Input: dimensioned drawing with shaded views. Units: mm. Origin: part minimum x, y, z. Give positions to 0.01 mm unless a question says otherwise; leave off trailing zeros. Write each loop counter-clockwise with the first axis right and the second up, starting at its lowest first coordinate (ties: lowest second). Pieces come first, ordered by that corner, then holes. Notation, with made-up numbers: M 79.25,83.5 L 114.25,83.5 A29 ccw 114.25,118.5 Z; hole C 58,68 d6. An arc over 180 degrees is marked long. Use CSV: the item, a comma, the result in double quotes. Start each with the question number.
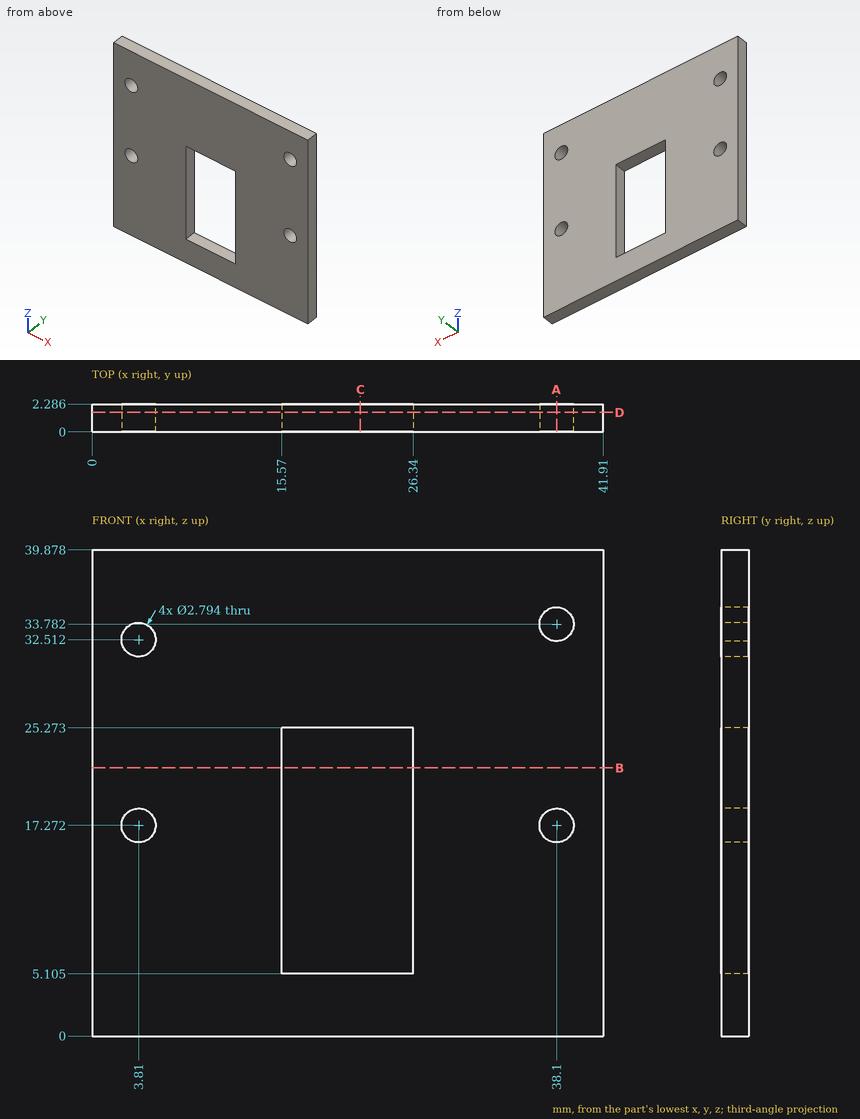
Q1. Section B-B, the plane z = 22. Return the cut outline in (x, y).
Q2. Material intervals for L1, parallel to Z at x = 38, y = 1.35 (1 decimal); L2, parallel to X at y = 0.4, z = 10.5; L3, parallel to Z at x = 16, y = 0.7 (1 decimal), sorted ascending. Write a range as [from, to].
Q3. Section D-D, the plane y = 1.6. Return the cut outline in (x, z) (1 decimal), and give its area (3 significant figures).
Q4. Section C-C, the plane x = 22. Return the cut outline in (y, z) (1 decimal).
Q5. Section A-A, the plane x = 38.1. Return the cut outline in (y, z) (1 decimal).
Check result:
1,outline,"M 0,0 L 15.57,0 L 15.57,2.29 L 0,2.29 Z; M 26.34,0 L 41.91,0 L 41.91,2.29 L 26.34,2.29 Z"
2,L1,"z = [0, 15.9], [18.7, 32.4], [35.2, 39.9]"
2,L2,"x = [0, 15.57], [26.34, 41.91]"
2,L3,"z = [0, 5.1], [25.3, 39.9]"
3,outline,"M 0,0 L 41.9,0 L 41.9,39.9 L 0,39.9 Z; hole C 3.8,17.3 d2.8; hole C 3.8,32.5 d2.8; hole M 15.6,5.1 L 26.3,5.1 L 26.3,25.3 L 15.6,25.3 Z; hole C 38.1,17.3 d2.8; hole C 38.1,33.8 d2.8"
3,area,"1,430 mm²"
4,outline,"M 0,0 L 2.3,0 L 2.3,5.1 L 0,5.1 Z; M 0,25.3 L 2.3,25.3 L 2.3,39.9 L 0,39.9 Z"
5,outline,"M 0,0 L 2.3,0 L 2.3,15.9 L 0,15.9 Z; M 0,18.7 L 2.3,18.7 L 2.3,32.4 L 0,32.4 Z; M 0,35.2 L 2.3,35.2 L 2.3,39.9 L 0,39.9 Z"
